CAD build for the part. Positions are in the model's coordinates, mm. Face numbers are marked on the shaded views. A direction names the side the tool comes from. Round coordinates to 2 decimals unless told otherwise and drop trailing zeros. Loops run counter-clockwise (first coordinate to the right, second up) from the corner with the lowest first, then second, coordinate; pieces in that order, holes last. Notation, with made-up numbers: M -17,69 L -6,69 A14 ccw -6,75 Z; hole C 47,78 d4. An arc over 180 degrees is marked long. Use one line per item in the form item = value.
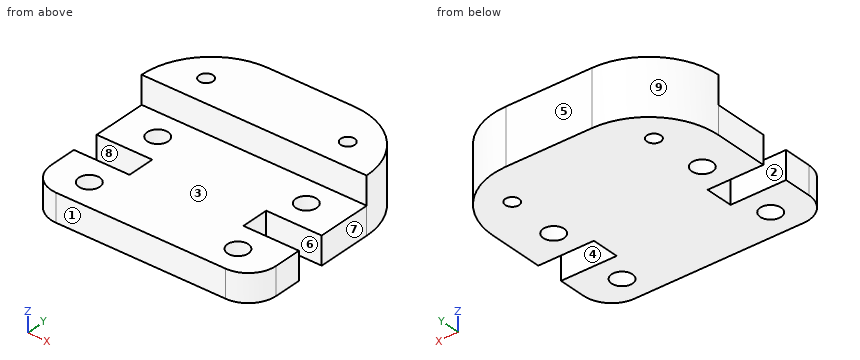
from build123d import *

# Parameters (mm, degrees)
SKETCH2_R           = 0.75
SKETCH2_R_2         = 0.5
BOSS_EXTRUDE1_DEPTH = 4
SKETCH3_W           = 16.2
SKETCH3_H           = 9.945
CUT_EXTRUDE2_DEPTH  = 2


with BuildPart() as part:
    # Sketch2 → Boss-Extrude1 (new body)
    with BuildSketch(Plane.XY):
        with BuildLine():
            Line((0, 9.945), (0, 6))
            Line((0, 6), (4, 6))
            Line((4, 6), (4, 4))
            Line((4, 4), (0, 4))
            Line((0, 4), (0, 2))
            ThreePointArc((0, 2), (0.585786438, 0.585786438), (2, 0))
            Line((2, 0), (14.2, 0))
            ThreePointArc((14.2, 0), (15.614213562, 0.585786438), (16.2, 2))
            Line((16.2, 2), (16.2, 4))
            Line((16.2, 4), (12.2, 4))
            Line((12.2, 4), (12.2, 6))
            Line((12.2, 6), (16.2, 6))
            Line((16.2, 6), (16.2, 9.945))
            ThreePointArc((16.2, 9.945), (14.735533906, 13.480533906), (11.2, 14.945))
            Line((11.2, 14.945), (5, 14.945))
            ThreePointArc((5, 14.945), (1.464466094, 13.480533906), (0, 9.945))
        make_face()
        with Locations((13.45, 8)):
            Circle(SKETCH2_R, mode=Mode.SUBTRACT)
        with Locations(Location((13.45, 2, 0), (0, 0, 180))):
            Circle(SKETCH2_R, mode=Mode.SUBTRACT)
        with Locations(Location((13.2, 11.942, 0), (0, 0, 180))):
            Circle(SKETCH2_R_2, mode=Mode.SUBTRACT)
        with Locations((3, 11.942)):
            Circle(SKETCH2_R_2, mode=Mode.SUBTRACT)
        with Locations((2.75, 2)):
            Circle(SKETCH2_R, mode=Mode.SUBTRACT)
        with Locations(Location((2.75, 8, 0), (0, 0, 180))):
            Circle(SKETCH2_R, mode=Mode.SUBTRACT)
    extrude(amount=BOSS_EXTRUDE1_DEPTH)

    # Sketch3 → Cut-Extrude2 (cut)
    with BuildSketch(Plane(origin=(0, 0, 4), x_dir=(-1, 0, 0), z_dir=(0, 0, -1))):
        with Locations((-8.1, 4.9725)):
            Rectangle(SKETCH3_W, SKETCH3_H)
    extrude(amount=CUT_EXTRUDE2_DEPTH, mode=Mode.SUBTRACT)


solid = part.part
1. Cut at A-A on y = 8. Write the cut outline in (x, z).
Completed:
outline = M 0,0 L 2,0 L 2,2 L 0,2 Z; M 3.5,0 L 12.7,0 L 12.7,2 L 3.5,2 Z; M 14.2,0 L 16.2,0 L 16.2,2 L 14.2,2 Z
2. Cut at B-B on x = 3. Write the cut outline in (y, z) (3 decimals).
Completed:
outline = M 0,0 L 1.293,0 L 1.293,2 L 0,2 Z; M 2.707,0 L 4,0 L 4,2 L 2.707,2 Z; M 6,0 L 7.293,0 L 7.293,2 L 6,2 Z; M 8.707,0 L 11.442,0 L 11.442,4 L 9.945,4 L 9.945,2 L 8.707,2 Z; M 12.442,0 L 14.528,0 L 14.528,4 L 12.442,4 Z
3. Pull direction Y, two halves, no side cores. Call the marked faces 6, 7, 8 and 9: +Y half, -Y half, draft (parallel to the pull), parting line (faces both ways), or undercut.
Completed:
face_6 = undercut
face_7 = draft
face_8 = undercut
face_9 = +Y half
4. Cut at D-D on x = 15. Write the cut outline in (y, z) (3 decimals).
Completed:
outline = M 0.167,0 L 4,0 L 4,2 L 0.167,2 Z; M 6,0 L 13.195,0 L 13.195,4 L 9.945,4 L 9.945,2 L 6,2 Z
5. Cut at C-C on z = 1.3. Write the cut outline in (x, y) (3 decimals), and give its area (3 significant figures).
Completed:
outline = M 0,2 A2 ccw 2,0 L 14.2,0 A2 ccw 16.2,2 L 16.2,4 L 12.2,4 L 12.2,6 L 16.2,6 L 16.2,9.945 A5 ccw 11.2,14.945 L 5,14.945 A5 ccw 0,9.945 L 0,6 L 4,6 L 4,4 L 0,4 Z; hole C 2.75,2 d1.5; hole C 2.75,8 d1.5; hole C 3,11.942 d1; hole C 13.45,2 d1.5; hole C 13.45,8 d1.5; hole C 13.2,11.942 d1
area = 205 mm2
6. Probe line 1 along X through (y, z) = (2, 0.4); line 2 along Y through (x, z) = (2.75, 1.3); line 3 along Y through (x, z) = (3, 1.75). List the from-to ranges inside material, lowest first. Write a range as from..to.
Completed:
line_1 = 0..2, 3.5..12.7, 14.2..16.2
line_2 = 0..1.25, 2.75..4, 6..7.25, 8.75..11.51, 12.38..14.41
line_3 = 0..1.29, 2.71..4, 6..7.29, 8.71..11.44, 12.44..14.53
7. Drop flat-ended pins along their axis: P1, Ø1.5, axis at x = 5.5, y = 9, coming from the +Z side; P2, Ø1, axis at x = 1, z = 1, coming from the -Y side; P3, Ø0.6, axis at x = 1.5, z = 0.5, coming from the +Y side. Give the stop position or say it passes through.
Completed:
P1 = 2
P2 = 0.06
P3 = 13.79
8. Tool access for the marked faces 1, 2, 3, 4 and 5: list every direction of +Z, -Z, +X, -X, +Y, -Y with a clear straight run to the whole face (end or side of a thin tool).
Completed:
face_1 = +Z, -Z, +X, -X, -Y
face_2 = +Z, -Z, -X
face_3 = +Z, +X, -X, -Y
face_4 = +Z, -Z, +X
face_5 = +Z, -Z, +X, -X, +Y
